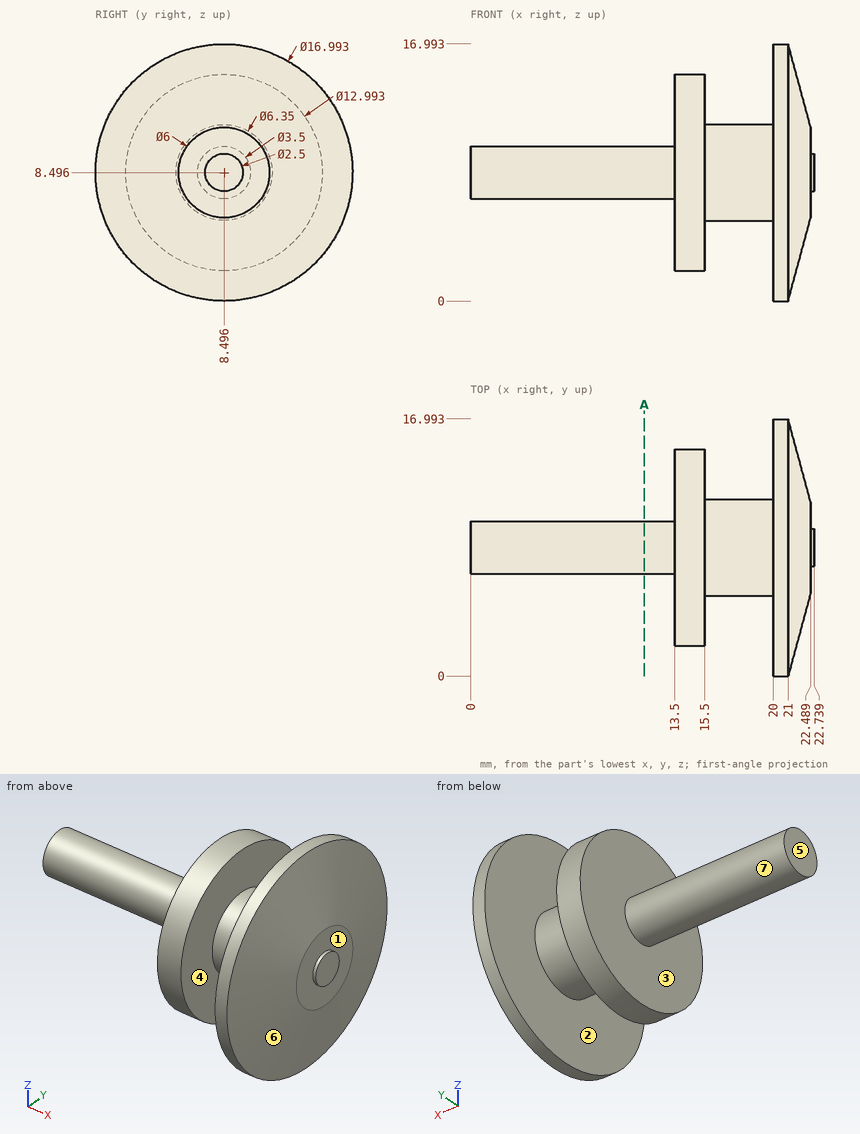
Answer from the drawing. Dimensions are ordinates in mm from the lowest x, y and z of the part. A direction names the side the tool comes from. Round coordinates to 2 decimals unless told otherwise and drop trailing zeros. Order: outer loops, then holes, each group sorted by start corner. A loop starts at its lowest first (then second) coordinate and runs counter-clockwise, first axis right, second up.
1) The part is cut by section A-A on x = 11.5. Write down the section's boundary in (y, z).
2) Flat-ended cylindrical pins translate along their axes: pin 1 (2 mm diameter, centred on y = 9.5, z = 14.5, fed in from +X); pin 2 (8 mm diameter, centred on x = 14.5, y = 6, fed in from +Z); pin 3 (1 mm diameter, centred on y = 3, z = 13, fed in from +X). Find the tip coordinate at first contact, or state that the pin passes through.
3) The mould has two halves that part along X. Classify the marked faces 4, 5, 6 and 7: released by +X, released by -X, zero draft, split by the parting line, or undercut.
4) For the marked faces 1, 2 and 3, determine the directions among +Z, -Z, +X, -X, +Y, -Y from which every point of the face is accessible in a straight line to the end or side of a thin tool.
5) Straight lines are drawn through the part: L1, parallel to X at y = 10, z = 10.25; L2, parallel to X at y = 6.25, z = 6; L3, parallel to X at y = 8.75, z = 14.25. For each, find the intervals that lie inside material, in ascending order.
Resolved:
1. outline: circle Ø3.5 at (8.5, 8.5)
2. pin 1: stops at x = 21.92
2. pin 2: stops at z = 14.99
2. pin 3: stops at x = 21.51
3. face 4: undercut
3. face 5: released by -X
3. face 6: released by +X
3. face 7: zero draft
4. face 1: +X
4. face 2: none
4. face 3: -X
5. L1: x = 13.5 to 22.49
5. L2: x = 13.5 to 15.5, 20 to 22.39
5. L3: x = 13.5 to 15.5, 20 to 21.74
